```python
from build123d import *

# Parameters (mm, degrees)
SKETCH2_W           = 28
SKETCH2_H           = 35.2
SKETCH2_R           = 11
BOSS_EXTRUDE3_DEPTH = 8
SKETCH3_W           = 10
SKETCH3_H           = 3
BOSS_EXTRUDE4_DEPTH = 28
BOSS_EXTRUDE5_DEPTH = 3
BOSS_EXTRUDE6_START = -28
BOSS_EXTRUDE6_DEPTH = 3
SKETCH4_R           = 2
CUT_EXTRUDE1_DEPTH  = 101.089134132
SKETCH2_3_R         = 11
SKETCH2_3_R_2       = 4.5
BOSS_EXTRUDE7_DEPTH = 0.5


with BuildPart() as part:
    # Sketch2 → Boss-Extrude3 (new body)
    with BuildSketch(Plane.XY.offset(-2.538447986)):
        with Locations((-78.732107824, 19.43595021)):
            Rectangle(SKETCH2_W, SKETCH2_H)
        with Locations((-78.732107824, 18.03595021)):
            Circle(SKETCH2_R, mode=Mode.SUBTRACT)
    extrude(amount=-BOSS_EXTRUDE3_DEPTH)

    # Sketch3 → Boss-Extrude4 (add)
    with BuildSketch(Plane.ZY.offset(92.732107824)):
        with Locations((-14.538447986, 3.33595021)):
            Rectangle(SKETCH3_W, SKETCH3_H)
    extrude(amount=-BOSS_EXTRUDE4_DEPTH)

    # Sketch3<3> → Boss-Extrude5 (add)
    with BuildSketch(Plane.ZY.offset(92.732107824)):
        Polygon((-19.538447986, 4.83595021), (-9.538447986, 4.83595021), (-9.538447986, 24.83595021), align=None)
    extrude(amount=-BOSS_EXTRUDE5_DEPTH)

    # Sketch3<4> → Boss-Extrude6 (add)
    with BuildSketch(Plane.ZY.offset(92.732107824).offset(BOSS_EXTRUDE6_START)):
        Polygon((-19.538447986, 4.83595021), (-9.538447986, 4.83595021), (-9.538447986, 24.83595021), (-10.538447986, 22.83595021), align=None)
    extrude(amount=BOSS_EXTRUDE6_DEPTH)

    # Sketch4 → Cut-Extrude1 (cut, through all)
    with BuildSketch(Plane(origin=(0, 4.83595021, 0), x_dir=(1, 0, 0), z_dir=(0, 1, 0))):
        with Locations(Location((-72.732107824, 15.038447986, 0), (0, 0, 270))):
            Circle(SKETCH4_R)
        with Locations(Location((-84.732107824, 15.038447986, 0), (0, 0, 90))):
            Circle(SKETCH4_R)
    extrude(amount=-CUT_EXTRUDE1_DEPTH, mode=Mode.SUBTRACT)

    # Sketch2<3> → Boss-Extrude7 (add)
    with BuildSketch(Plane.XY.offset(-2.538447986)):
        with Locations((-78.732107824, 18.03595021)):
            Circle(SKETCH2_3_R)
        with Locations((-78.732107824, 18.03595021)):
            Circle(SKETCH2_3_R_2, mode=Mode.SUBTRACT)
    extrude(amount=-BOSS_EXTRUDE7_DEPTH)


solid = part.part
```
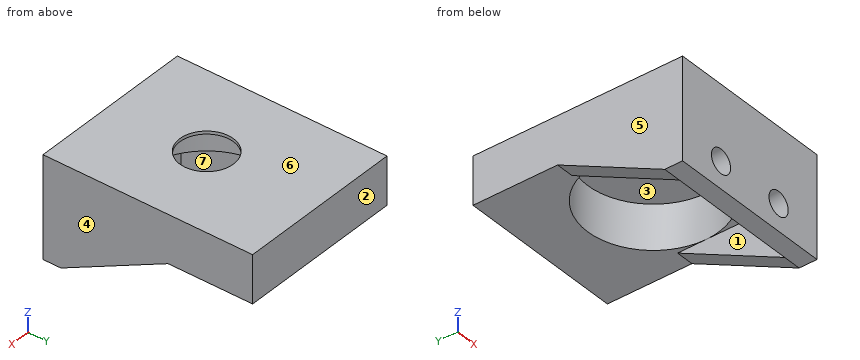
Work out the finished part from the listing and answer in its coordinate system (mm). Face numbers are marked on the shaded views. A direction names the side the tool comes from. Coordinates: 2 decimals unless noted, no trailing zeros. Order: outer loops, then holes, each group sorted by start corner. A loop starts at its lowest first (then second) coordinate and runs counter-clockwise, first axis right, second up. Notation, with made-up numbers: (-12, -34) - (7, -34) arc R15 cw to (7, -16) - close; hole circle Ø9 at (89, -34). An arc over 180 degrees is marked (long way). Answer as a JSON object with one key per item and string values.
1. Each of these flat-tipped pins is pushed along its axis until it touches: P1, Ø2, axis at x = -69, y = 29.5, coming from the -Z side; P2, Ø4.5, axis at x = -80.5, z = -16, coming from the +Y side; P3, Ø6.5, axis at x = -81.5, y = 15, coming from the -Z side. Where does it stop, or does it pass through?
Output values:
{"P1": "stops at z = -10.54", "P2": "stops at y = 4.84", "P3": "stops at z = -3.04"}
2. Find section A-A on z = -4.75. Determine the outline of the cut face in (x, y).
Output values:
{"outline": "(-92.73, 1.84) - (-64.73, 1.84) - (-64.73, 37.04) - (-92.73, 37.04) - close; hole circle Ø22 at (-78.73, 18.04)"}
3. Consider line 1 (X direction, y = 7, z = -14); line 2 (Z direction, x = -88.5, y = 25.5); line 3 (Z direction, x = -82.25, y = 22). Determine where each line is inside the solid, lowest interval first.
Output values:
{"line 1": "x = -92.73 to -89.73, -67.73 to -64.73", "line 2": "z = -10.54 to -2.54", "line 3": "z = -3.04 to -2.54"}
4. Find section D-D on x = -90.25. Determine the outline of the cut face in (y, z), plus the area to 3 significant figures.
Output values:
{"outline": "(1.84, -19.54) - (4.84, -19.54) - (22.84, -10.54) - (37.04, -10.54) - (37.04, -2.54) - (1.84, -2.54) - close", "area": "390 mm²"}
5. Find section B-B on x = -76.5. Determine the outline of the cut face in (y, z).
Output values:
{"outline": "(1.84, -19.54) - (4.84, -19.54) - (4.84, -10.54) - (7.26, -10.54) - (7.26, -3.04) - (14.13, -3.04) - (14.13, -2.54) - (1.84, -2.54) - close; (21.94, -3.04) - (28.81, -3.04) - (28.81, -10.54) - (37.04, -10.54) - (37.04, -2.54) - (21.94, -2.54) - close"}
6. A tool of negligible diameter and unlimited length cuts with its end or side. For the marked faces 1, 2 and 3, from which of +Z, -Z, +X, -X, +Y, -Y can it reach the whole face along a straight path? Write none if from no direction.
Output values:
{"face 1": "-Z, +Y", "face 2": "+Z, -Z, +X, -X, +Y", "face 3": "-Z"}
7. Find section C-C on y = 19. Determine the outline of the cut face in (x, z), plus the area to 3 significant figures.
Output values:
{"outline": "(-92.73, -12.46) - (-89.73, -12.46) - (-89.73, -10.54) - (-89.69, -10.54) - (-89.69, -3.04) - (-83.13, -3.04) - (-83.13, -2.54) - (-92.73, -2.54) - close; (-74.34, -3.04) - (-67.77, -3.04) - (-67.77, -10.54) - (-67.73, -10.54) - (-67.73, -12.46) - (-64.73, -12.46) - (-64.73, -2.54) - (-74.34, -2.54) - close", "area": "66.7 mm²"}
8. The mould has two halves that part along X. Classify the marked faces 4, 5, 6 and 7: +X half, -X half, draft (parallel to the pull), parting line (faces both ways), or undercut.
Output values:
{"face 4": "+X half", "face 5": "-X half", "face 6": "draft", "face 7": "undercut"}
